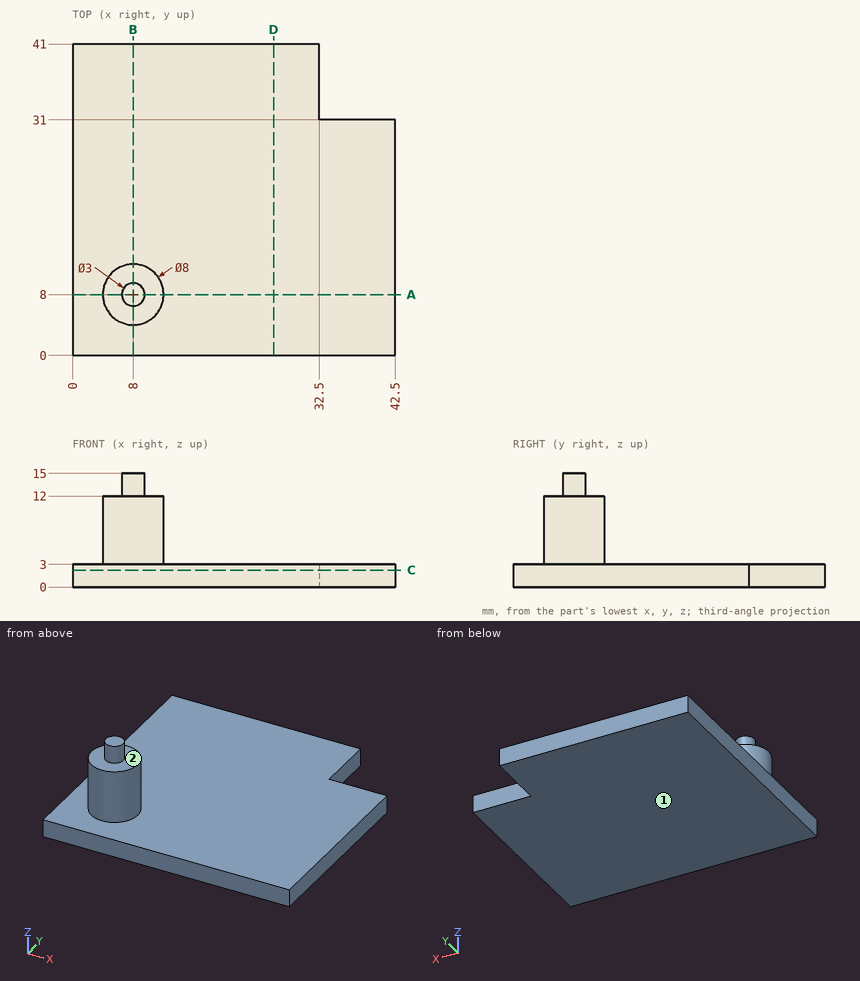
Could you check a few things on this drawing? It's one solid part, dimensions in mm from its lowest x, y, z. A direction names the side the tool comes from. Coordinates: 2 decimals unless noted, no trailing zeros. Write each loop counter-clockwise with the first axis right and the second up, starting at its lowest first coordinate (ties: lowest second). Pieces come first, ordered by that corner, then holes. Notation, with made-up numbers: (-20, 36.5) - (-1, 36.5) arc R13 ccw to (-1, 53.5) - close; hole circle Ø6 at (20, 25.5). An arc over 180 degrees is marked (long way). Return JSON: item names as keys, results as strings. Group by question number.
Item 1: I'm going to push flat-ended pins straight in: pin 1 Ø4 at (x, z) = (37, 4.5) entering from +Y; pin 2 Ø1 at (y, z) = (4.5, 12) entering from -X; pin 3 Ø1.5 at (y, z) = (36.5, 1) entering from +X. Where does each tip first touch, or does it pass through?
Item 2: If we section it at A-A (y = 8): Write out the boundary of the cut face in (x, z).
Item 3: If we section it at D-D (x = 26.5): Write out the boundary of the cut face in (y, z), then the cut area to 3 significant figures.
Item 4: Which directions (+Z, -Z, +X, -X, +Y, -Y) give clear straight access to the entire face, cutting with the end or side of a thin tool? Please do the marked faces 1 and 2.
Item 5: Please list where these lines run through material, in increasing order: probe 1 along Z at (x, y) = (25.5, 26); probe 2 along Z at (x, y) = (9.5, 7); probe 3 along Y at (x, z) = (9.5, 4.25).
Item 6: If we section it at C-C (z = 2.25): Write out the boundary of the cut face in (x, y).
Item 7: If we section it at B-B (x = 8): Write out the boundary of the cut face in (y, z).
Return value:
{
 "1": {"pin 1": "stops at y = 31", "pin 2": "stops at x = 5.35", "pin 3": "stops at x = 32.5"},
 "2": {"outline": "(0, 0) - (42.5, 0) - (42.5, 3) - (12, 3) - (12, 12) - (9.5, 12) - (9.5, 15) - (6.5, 15) - (6.5, 12) - (4, 12) - (4, 3) - (0, 3) - close"},
 "3": {"outline": "(0, 0) - (41, 0) - (41, 3) - (0, 3) - close", "area": "123 mm^2"},
 "4": {"face 1": "-Z, +X, -X, +Y, -Y", "face 2": "+Z"},
 "5": {"probe 1": "z = 0 to 3", "probe 2": "z = 0 to 12", "probe 3": "y = 4.29 to 11.71"},
 "6": {"outline": "(0, 0) - (42.5, 0) - (42.5, 31) - (32.5, 31) - (32.5, 41) - (0, 41) - close"},
 "7": {"outline": "(0, 0) - (41, 0) - (41, 3) - (12, 3) - (12, 12) - (9.5, 12) - (9.5, 15) - (6.5, 15) - (6.5, 12) - (4, 12) - (4, 3) - (0, 3) - close"}
}
